Geometry: final body of the model. Coordinates: model frame, mm. Face numbers are marked on the shaded views. A direction names the side the tool comes from. Round coordinates to 2 decimals unless told otherwise and drop trailing zeros. Loops run counter-clockwise (first coordinate to the right, second up) from the corner with the lowest first, then second, coordinate; pieces in that order, holes last. Notation, with made-up numbers: (-17, 45.5) - (27, 45.5) arc R16 cw to (27, 62.5) - close; hole circle Ø5 at (38, 58). An arc over 180 degrees is marked (long way). Answer as a JSON object with one key per item and string values. Group by question number.
Item 1: Section A-A (y = 0). Return the cut outline in (x, z).
Item 2: First-contact query: pin 1 (5 mm diameter, centred on y = -8, z = -1.5, fed in from +X); pin 2 (2.5 mm diameter, centred on x = -15, y = -14.5, fed in from -Z); pin 3 (3 mm diameter, centred on x = -3.5, y = 0.5, fed in from +Z); pin 4 (0.7 mm diameter, centred on x = 13.5, y = 13.5, fed in from -Z). Flat tips, straight axial feed; report the tip coordinate or a pass-through.
Item 3: Draft query along Y for the marked faces 1, 2, 3 and 4. Return one class per face: released by +Y, released by -Y, zero draft, split by the parting line, or undercut.
Item 4: Line query: line 1 (Y direction, x = 13.75, z = -6.25); line 2 (X direction, y = -15.5, z = -7.5); line 3 (Y direction, x = 25.4, z = -5.5). Output: solid intervals per line, ascending.
Item 5: Section B-B (y = 13.75). Return the cut outline in (x, z).
Item 6: Section D-D (z = -5). Count the separate pieces of the cut face and the enclosed holes in it, plus the area to 3 significant figures.
Item 7: Section C-C (x = -3). Return the cut outline in (y, z).
Item 8: Reachability of the marked faces 5, 6, 7 and 8 from +Z, -Z, +X, -X, +Y, -Y: full face, straight path, thin tool, end or side. Return the list, or none.
Autodesk Inventor part; units mm, degrees
ref_plane "YZ Plane" through (0, 0, 0) normal (1, 0, 0) x (0, 1, 0)
ref_plane "XZ Plane" through (0, 0, 0) normal (0, 1, 0) x (-1, 0, 0)
ref_plane "XY Plane" through (0, 0, 0) normal (0, 0, 1) x (1, 0, 0)
sketch "Sketch1" plane through (0, 0, 0) normal (0, 0, 1) x (1, 0, 0)
  circle A0 centre (0, 0) radius 25.4 construction
  line L0 (-13.75, -13.75) -> (13.75, -13.75) construction
  line L1 (13.75, -13.75) -> (13.75, 13.75) construction
  line L2 (13.75, 13.75) -> (-13.75, 13.75) construction
  line L3 (-13.75, 13.75) -> (-13.75, -13.75) construction
  line L4 (-13.75, -13.75) -> (13.75, 13.75) construction
  line L5 (13.75, -13.75) -> (-13.75, 13.75) construction
  circle A1 centre (0, 0) radius 7.25
  circle A2 centre (-13.75, 13.75) radius 1.2
  circle A3 centre (-13.75, 13.75) radius 2.7
  circle A4 centre (-25.4, 0) radius 1.7
  circle A5 centre (-25.4, 0) radius 5
  line L6 (-17, 17) -> (17, 17)
  line L7 (17, 17) -> (17, -17)
  line L8 (17, -17) -> (-17, -17)
  line L9 (-17, -17) -> (-17, 17)
  line L10 (-17, 17) -> (17, -17) construction
  line L11 (17, 17) -> (-17, -17) construction
  line L12 (-25.4, 5) -> (-18, 5)
  line L13 (-25.4, -5) -> (-18, -5)
  line L14 (0, 17) -> (0, -17) construction
  line L15 (-17, 0) -> (17, 0) construction
  circle A6 centre (25.4, 0) radius 1.7
  circle A7 centre (25.4, 0) radius 5
  line L16 (25.4, 5) -> (18, 5)
  line L17 (25.4, -5) -> (18, -5)
  circle A8 centre (13.75, 13.75) radius 1.2
  circle A9 centre (13.75, 13.75) radius 2.7
  circle A10 centre (-13.75, -13.75) radius 1.2
  circle A11 centre (-13.75, -13.75) radius 2.7
  circle A12 centre (13.75, -13.75) radius 2.7
  circle A13 centre (13.75, -13.75) radius 1.2
  line L18 (-18, 18) -> (18, 18)
  line L19 (18, 18) -> (18, -18)
  line L20 (18, -18) -> (-18, -18)
  line L21 (-18, -18) -> (-18, 18)
  line L22 (-18, 18) -> (18, -18) construction
  line L23 (18, 18) -> (-18, -18) construction
  circle A14 centre (-13.75, 13.75) radius 12 construction
  line L24 (-1.75, 13.75) -> (-1.75, 15.25) construction
  line L25 (-1.75, 13.75) -> (-1.75, 10.15) construction
  line L26 (-11.35, 13.75) -> (-11.35, 10.15) construction
  line L27 (-11.35, 13.75) -> (-11.35, 15.25) construction
  line L28 (-11.35, 10.15) -> (-1.75, 10.15)
  line L29 (-1.75, 10.15) -> (-1.75, 15.25)
  line L30 (-1.75, 15.25) -> (-11.35, 15.25)
  line L31 (-11.35, 15.25) -> (-11.35, 10.15)
  point P0 (-17, 3.8)
  point P1 (-17, -3.8)
  point P2 (17, 3.8)
  point P3 (17, -3.8)
  dimension "d22" = 24
  dimension "d0" = 50.8
  dimension "d1" = 27.5
  dimension "d2" = 27.5
  dimension "d3" = 14.5
  dimension "d4" = 2.4
  dimension "d5" = 5.4
  dimension "d6" = 3.4
  dimension "d7" = 10
  dimension "d8" = 34
  dimension "d9" = 34
  dimension "d10" = 36
  dimension "d11" = 36
  dimension "d24" = 1.5
  dimension "d25" = 3.6
extrude "Extrusion1" add sketch "Sketch1" against normal blind 9.2 contours L21 L18 L19 L20
extrude "Extrusion3" add sketch "Sketch1" against normal blind 7.4 contours A3 L31 | L31 A3 | A9 | A11 | A12
extrude "Extrusion4" add sketch "Sketch1" against normal blind 2.2 contours A1 | A2 | A3 L31 L30 L29 L28 | L6 L7 L8 L9 | A8 | A10 | A13
extrude "Extrusion5" add sketch "Sketch1" against normal blind 8.65 contours A5 | A5 L12 L21 L13 | L16 A7 L17 L19 | A7
extrude "Extrusion6" cut sketch "Sketch1" along normal mid plane 22 contours A3 L31 | A3 L31 L30 L29 L28 picked at (-11.2949, 13.4692)
fillet "Fillet1" radius 0.6 10 edges at (-18, -18, -4.6) (-18, 18, -4.6) (18, 18, -4.6) (18, -18, -4.6) (-30.4, 0, -8.65) (-21.7, 5, -8.65) (-21.7, -5, -8.65) (30.4, 0, -8.65) (21.7, 5, -8.65) (21.7, -5, -8.65)
equation "\"d9\" = d8"
properties part number "cameraBottom"
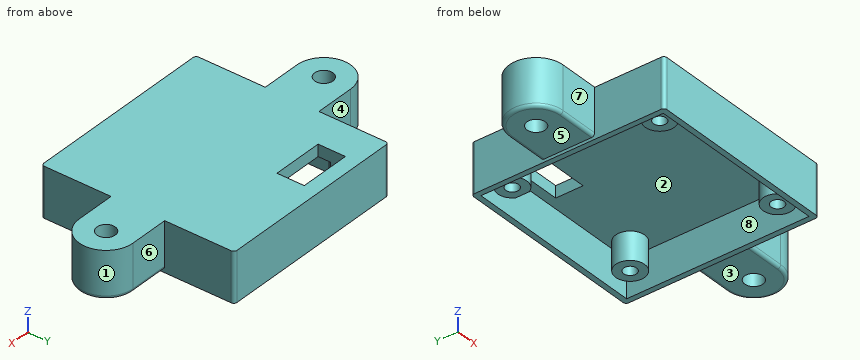
Values:
{
 "1": {"outline": "(-30.4, -8.05) arc R0.6 ccw to (-29.8, -8.65) - (-27.1, -8.65) - (-27.1, 0) - (-30.4, 0) - close; (-23.7, -8.65) - (-18, -8.65) - (-18, -9.2) - (-17, -9.2) - (-17, -2.2) - (17, -2.2) - (17, -9.2) - (18, -9.2) - (18, -8.65) - (23.7, -8.65) - (23.7, 0) - (-23.7, 0) - close; (27.1, -8.65) - (29.8, -8.65) arc R0.6 ccw to (30.4, -8.05) - (30.4, 0) - (27.1, 0) - close"},
 "2": {"pin 1": "stops at x = 18", "pin 2": "stops at z = -7.4", "pin 3": "stops at z = 0", "pin 4": "stops at z = -2.2"},
 "3": {"face 1": "split by the parting line", "face 2": "undercut", "face 3": "zero draft", "face 4": "released by +Y"},
 "4": {"line 1": "y = -18 to -17, -16.45 to -14.95, -12.55 to -11.05, 11.05 to 12.55, 14.95 to 16.45, 17 to 18", "line 2": "x = -18 to -17, 17 to 18", "line 3": "y = -5 to -1.7, 1.7 to 5"},
 "5": {"outline": "(-18, -9.2) - (-17, -9.2) - (-17, -2.2) - (-16.45, -2.2) - (-16.45, -7.4) - (-14.95, -7.4) - (-14.95, -2.2) - (-12.55, -2.2) - (-12.55, -7.4) - (-11.35, -7.4) - (-11.35, 0) - (-18, 0) - close; (-1.75, -2.2) - (11.05, -2.2) - (11.05, -7.4) - (12.55, -7.4) - (12.55, -2.2) - (14.95, -2.2) - (14.95, -7.4) - (16.45, -7.4) - (16.45, -2.2) - (17, -2.2) - (17, -9.2) - (18, -9.2) - (18, 0) - (-1.75, 0) - close"},
 "6": {"separate pieces": "5", "enclosed holes": "7", "area": "421 mm^2"},
 "7": {"outline": "(-18, -9.2) - (-17, -9.2) - (-17, -2.2) - (10.15, -2.2) - (10.15, 0) - (-18, 0) - close; (15.25, -2.2) - (17, -2.2) - (17, -9.2) - (18, -9.2) - (18, 0) - (15.25, 0) - close"},
 "8": {"face 5": "-Z, -X, +Y, -Y", "face 6": "+Z, -Z, +X, +Y", "face 7": "+Z, -Z, -X, -Y", "face 8": "-Z"}
}
